Verification items for the finished model (mm, model axes). Face numbers are marked on the shaded views. A direction names the side the tool comes from. Round coordinates to 2 decimals unless told otherwise and drop trailing zeros. Write each loop counter-clockwise with the first axis right and the second up, starting at its lowest first coordinate (ties: lowest second). Pieces come first, ordered by that corner, then holes. Notation, with made-up numbers: (77, 1) - (110, 1) arc R31 cw to (110, 40) - close; hole circle Ø6 at (79, 53). An arc over 180 degrees is marked (long way). Write each question's results on one line, items separated by ' | '.
```python
from build123d import *

# Parameters (mm, degrees)
SKETCH1_R                    = 14.975
EXTRUDE1_DEPTH               = 27
EXTRUDE2_DEPTH               = 2
SKETCH3_R                    = 1.5
EXTRUDE3_DEPTH               = 3
EXTRUDE6_DEPTH               = 3
CIRPATTERN1_COUNT            = 3
SKETCH5_W                    = 37.119401026
SKETCH5_H                    = 9.762697639
EXTRUDE7_DEPTH               = 11.5
SKETCH6_R                    = 2.5
EXTRUDE8_DEPTH               = 31.5
SKETCH7_R                    = 3.95
EXTRUDE9_DEPTH               = 28
F_4_0_4_DIAMETER_HOLE1_D     = 4
F_4_0_4_DIAMETER_HOLE1_DEPTH = 15
EXTRUDE10_DEPTH              = 4.8


with BuildPart() as part:
    # Sketch1 → Extrude1 (new body)
    with BuildSketch(Plane.XY):
        Circle(SKETCH1_R)
    extrude(amount=EXTRUDE1_DEPTH)

    # Sketch2 → Extrude2 (add)
    with BuildSketch(Plane.XY):
        with BuildLine():
            Line((-3.363320174, 17.968543962), (-4.221577642, 14.367634016))
            Line((-4.221577642, 14.367634016), (4.221577642, 14.367634016))
            Line((4.221577642, 14.367634016), (3.5, 17))
            ThreePointArc((3.5, 17), (0.489070236, 20.465661597), (-3.363320174, 17.968543962))
        make_face()
    extrude2 = extrude(amount=EXTRUDE2_DEPTH)

    # Sketch3 → Extrude3 (cut)
    with BuildSketch(Plane.XY.offset(2)):
        with Locations((0, 17)):
            Circle(SKETCH3_R)
    extrude3 = extrude(amount=-EXTRUDE3_DEPTH, mode=Mode.SUBTRACT)

    # Sketch4 → Extrude6 (cut, symmetric)
    with BuildSketch(Plane(origin=(0, 0, 0), x_dir=(0, 0, -1), z_dir=(1, 0, 0))):
        Polygon((-2, 14.975), (-2, 13.475), (-5.5, 13.475), (-10, 14.975), align=None)
    extrude6 = extrude(amount=EXTRUDE6_DEPTH, both=True, mode=Mode.SUBTRACT)

    # CirPattern1: Extrude2, Extrude3, Extrude6 ×3 about axis
    cirpattern1_axis = Axis((0, 0, 0), (0, 0, 1))
    for i in range(1, CIRPATTERN1_COUNT):
        add(extrude2.rotate(cirpattern1_axis, i * 360 / CIRPATTERN1_COUNT))
        add(extrude3.rotate(cirpattern1_axis, i * 360 / CIRPATTERN1_COUNT), mode=Mode.SUBTRACT)
        add(extrude6.rotate(cirpattern1_axis, i * 360 / CIRPATTERN1_COUNT), mode=Mode.SUBTRACT)

    # Sketch5 → Extrude7 (cut)
    with BuildSketch(Plane.XY.offset(27)):
        with Locations((1.994416424, 14.88134882)):
            Rectangle(SKETCH5_W, SKETCH5_H)
    extrude7 = extrude(amount=-EXTRUDE7_DEPTH, mode=Mode.SUBTRACT)

    # Mirror2: Extrude7 across plane
    add(extrude7.mirror(Plane.ZX), mode=Mode.SUBTRACT)

    # Sketch6 → Extrude8 (cut, through all)
    with BuildSketch(Plane.XZ.offset(10)):
        with Locations((-6.545813687, 21)):
            Circle(SKETCH6_R)
        with Locations((6.454186313, 21)):
            Circle(SKETCH6_R)
    extrude(amount=-EXTRUDE8_DEPTH, mode=Mode.SUBTRACT)

    # Sketch7 → Extrude9 (cut, through all)
    with BuildSketch(Plane(origin=(0, 0, 0), x_dir=(-1, 0, 0), z_dir=(0, 0, -1))):
        Circle(SKETCH7_R)
    extrude(amount=-EXTRUDE9_DEPTH, mode=Mode.SUBTRACT)

    # 4.0 _4_ Diameter Hole1
    with Locations(Plane(origin=(-11.5, -0.00158702, 27), x_dir=(1, 0, 0), z_dir=(0, 0, 1))):
        with Locations((0, 0), (23, 0)):
            Hole(F_4_0_4_DIAMETER_HOLE1_D / 2, depth=F_4_0_4_DIAMETER_HOLE1_DEPTH)

    # Sketch9 → Extrude10 (add)
    with BuildSketch(Plane.XY):
        with BuildLine():
            Line((-7.482050917, 14.706084254), (-6.790528029, 13.346885558))
            ThreePointArc((-6.790528029, 13.346885558), (-13.855474408, 5.681237008), (-14.205824206, -4.737634814))
            Line((-14.205824206, -4.737634814), (-15.71367648, -5.032928718))
            ThreePointArc((-15.71367648, -5.032928718), (-15.22884108, 6.350779429), (-7.482050917, 14.706084254))
        make_face()
        with BuildLine():
            Line((7.482050917, 14.706084254), (6.790528029, 13.346885558))
            ThreePointArc((6.790528029, 13.346885558), (13.82132698, 5.763813452), (14.261351836, -4.567764094))
            Line((14.261351836, -4.567764094), (15.71367648, -5.032928718))
            ThreePointArc((15.71367648, -5.032928718), (15.22884108, 6.350779429), (7.482050917, 14.706084254))
        make_face()
    extrude(amount=EXTRUDE10_DEPTH)


solid = part.part
```
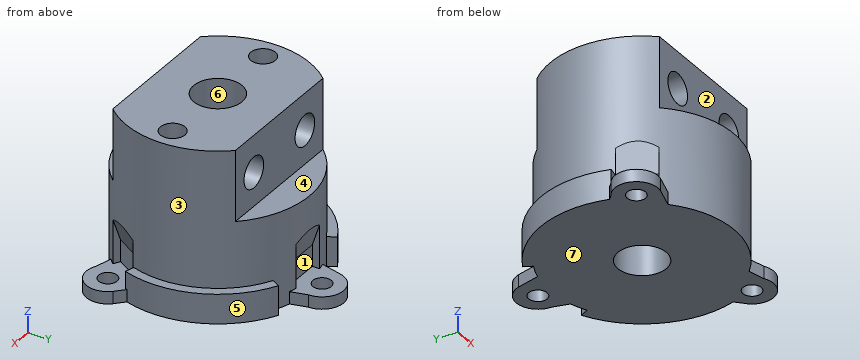
(1) Mould release check, pull along X, two halves, no side actions. Record for the marked faces 5, 6 and 7: released by +X, released by -X, zero draft, split by the parting line, or undercut.
Answer:
face 5: released by +X | face 6: undercut | face 7: zero draft
(2) Section check A-A (z = 23). Record the cut outline in (x, y) (3 decimals).
Answer:
outline: (-11.147, -10) - (-8.046, -10) - (-8.046, 10) - (-11.147, 10) arc R14.975 ccw to start; (-5.046, -10) - (4.954, -10) - (4.954, 10) - (-5.046, 10) - close; (7.954, -10) - (11.147, -10) arc R14.975 ccw to (11.147, 10) - (7.954, 10) - close; hole circle Ø4 at (-11.5, -0.002); hole circle Ø7.9 at (0, 0); hole circle Ø4 at (11.5, -0.002)
(3) Thickness scan on L1, parallel to Y at x = 0, z = 0.9 (3 decimals); L2, parallel to Y at x = 0, z = 16.25; L3, parallel to X at y = 11, z = 9.25. Record the ranges inside material, lowest first.
Answer:
L1: -14.975 to -3.95, 3.95 to 15.5, 18.5 to 20.5 | L2: -10 to -3.95, 3.95 to 10 | L3: -10.16 to 10.16
(4) Set-up check for the marked faces 1, 2, 3 and 4: record each of +Z, -Z, +X, -X, +Y, -Y from which the full face is reachable in a straight line by a thin tool's end or side.
Answer:
face 1: +Y | face 2: +Z, +X, -X, -Y | face 3: +Z | face 4: +Z, +X, -X, +Y
(5) Go/stop test with flat-tipped pins: pin 1 Ø4 at (x, z) = (8.5, 24) entering from -Y; pin 2 Ø3 at (x, y) = (11.5, 0) entering from +Z; pin 3 Ø3 at (x, z) = (-0.5, 4.5) entering from +Y. Record where each tip stops, or that it passes through.
Answer:
pin 1: y = -10 | pin 2: z = 12 | pin 3: y = 13.64
(6) Section check C-C (x = 0). Record the cut outline in (y, z) (3 decimals).
Answer:
outline: (-14.975, 0) - (-3.95, 0) - (-3.95, 27) - (-10, 27) - (-10, 15.5) - (-14.975, 15.5) - close; (3.95, 0) - (15.5, 0) - (15.5, 2) - (13.475, 2) - (13.475, 5.5) - (14.975, 10) - (14.975, 15.5) - (10, 15.5) - (10, 27) - (3.95, 27) - close; (18.5, 0) - (20.5, 0) - (20.5, 2) - (18.5, 2) - close
(7) Section check B-B (y = -1). Record the cut outline in (x, z).
Answer:
outline: (-16.47, 0) - (-3.82, 0) - (-3.82, 27) - (-9.77, 27) - (-9.77, 12) - (-13.23, 12) - (-13.23, 27) - (-14.94, 27) - (-14.94, 4.8) - (-16.47, 4.8) - close; (3.82, 0) - (16.47, 0) - (16.47, 4.8) - (14.94, 4.8) - (14.94, 27) - (13.23, 27) - (13.23, 12) - (9.77, 12) - (9.77, 27) - (3.82, 27) - close; hole circle Ø5 at (-6.55, 21); hole circle Ø5 at (6.45, 21)
(8) Section check D-D (y = -8.5). Record the cut outline in (x, z).
Answer:
outline: (-18.22, 0) - (-16.22, 0) - (-16.22, 2) - (-18.22, 2) - close; (-13.22, 0) - (13.22, 0) - (13.22, 2) - (10.65, 2) - (10.65, 5.5) - (12.33, 9.86) - (12.33, 27) - (-12.33, 27) - (-12.33, 9.86) - (-10.65, 5.5) - (-10.65, 2) - (-13.22, 2) - close; (16.22, 0) - (18.22, 0) - (18.22, 2) - (16.22, 2) - close; hole circle Ø5 at (-6.55, 21); hole circle Ø5 at (6.45, 21)
